Can you work these out from the model? Positions are in its coordinate system, mm. A direction names the side the tool comes from. Give positions to 0.01 mm unless a question says otherwise; leave off trailing zeros. Loops run counter-clockwise (first coordinate to the right, second up) from the corner with the lowest first, then second, coordinate; pieces in that order, holes last. Notation, with made-up numbers: (-39, -1) - (-25, -1) arc R30 cw to (-25, 38) - close; hole circle Ø1 at (-23, 28). An arc over 180 degrees is marked (long way). Answer as a JSON object with one key per item and string values.
```python
from build123d import *

# Parameters (mm, degrees)
SKETCH1_W           = 25.4
SKETCH1_H           = 50.8
SKETCH1_W_2         = 19.05
SKETCH1_H_2         = 44.45
BOSS_EXTRUDE1_DEPTH = 154.051
SKETCH2_R           = 3.175
CUT_EXTRUDE1_DEPTH  = 165.187425222
SKETCH3_R           = 3.175
CUT_EXTRUDE2_DEPTH  = 165.187425222


with BuildPart() as part:
    # Sketch1 → Boss-Extrude1 (new body)
    with BuildSketch(Plane.XY):
        with Locations((12.7, 25.4)):
            Rectangle(SKETCH1_W, SKETCH1_H)
        with Locations((12.7, 25.4)):
            Rectangle(SKETCH1_W_2, SKETCH1_H_2, mode=Mode.SUBTRACT)
    extrude(amount=BOSS_EXTRUDE1_DEPTH)

    # Sketch2 → Cut-Extrude1 (cut, through all)
    with BuildSketch(Plane(origin=(0, 50.8, 0), x_dir=(1, 0, 0), z_dir=(0, 1, 0))):
        with Locations(Location((12.7, -126.111, 0), (0, 0, 270))):
            Circle(SKETCH2_R)
        with Locations(Location((12.7, -107.061, 0), (0, 0, 270))):
            Circle(SKETCH2_R)
        with Locations(Location((12.7, -88.011, 0), (0, 0, 270))):
            Circle(SKETCH2_R)
        with Locations(Location((12.7, -27.94, 0), (0, 0, 90))):
            Circle(SKETCH2_R)
        with Locations(Location((12.7, -46.99, 0), (0, 0, 90))):
            Circle(SKETCH2_R)
        with Locations(Location((12.7, -66.04, 0), (0, 0, 90))):
            Circle(SKETCH2_R)
    extrude(amount=-CUT_EXTRUDE1_DEPTH, mode=Mode.SUBTRACT)

    # Sketch3 → Cut-Extrude2 (cut, through all)
    with BuildSketch(Plane(origin=(25.4, 0, 0), x_dir=(0, 0, -1), z_dir=(1, 0, 0))):
        with Locations(Location((-18.542, 25.4, 0), (0, 0, 90))):
            Circle(SKETCH3_R)
        with Locations(Location((-37.592, 25.4, 0), (0, 0, 90))):
            Circle(SKETCH3_R)
        with Locations(Location((-56.642, 25.4, 0), (0, 0, 90))):
            Circle(SKETCH3_R)
        with Locations(Location((-75.692, 25.4, 0), (0, 0, 90))):
            Circle(SKETCH3_R)
    extrude(amount=-CUT_EXTRUDE2_DEPTH, mode=Mode.SUBTRACT)


solid = part.part
```
1) Imagine slicing it at D-D on x = 12.7. Give the number of separate pieces and of enclosed holes in the cut face, and give its area (3 significant figures).
Check sheet entries:
{"separate pieces": "14", "enclosed holes": "0", "area": "736 mm2"}
2) If we mould it in two halves opening along X, with no side actions, what happens to faces 3 (the cylindrical face through (23.835, 27.107, 59.319)), 4 (the flat face through (13, 47.625, 76))? For each: released by +X, released by -X, zero draft, split by the parting line, or undercut.
Check sheet entries:
{"face 3": "zero draft", "face 4": "undercut"}
3) Imagine slicing it at C-C on z = 11.5. Write out the boundary of the cut face in (x, y) (3 decimals).
Check sheet entries:
{"outline": "(0, 0) - (25.4, 0) - (25.4, 50.8) - (0, 50.8) - close; hole (3.175, 3.175) - (22.225, 3.175) - (22.225, 47.625) - (3.175, 47.625) - close"}
4) I need wall thicknesses on L1, parallel to X at y = 40.5, z = 134 (3 decimals); L2, parallel to Y at x = 5.75, z = 7 (3 decimals). Which ranges of each line are inside material? Lowest first, please.
Check sheet entries:
{"L1": "0 to 3.175, 22.225 to 25.4", "L2": "0 to 3.175, 47.625 to 50.8"}
5) Imagine slicing it at A-A on z = 46.99. Write out the boundary of the cut face in (x, y) (3 decimals), and give its area (3 significant figures).
Check sheet entries:
{"outline": "(0, 0) - (9.525, 0) - (9.525, 3.175) - (3.175, 3.175) - (3.175, 47.625) - (9.525, 47.625) - (9.525, 50.8) - (0, 50.8) - close; (15.875, 0) - (25.4, 0) - (25.4, 50.8) - (15.875, 50.8) - (15.875, 47.625) - (22.225, 47.625) - (22.225, 3.175) - (15.875, 3.175) - close", "area": "403 mm2"}
6) Imagine slicing it at B-B on y = 39.5. Write out the boundary of the cut face in (x, z) (3 decimals).
Check sheet entries:
{"outline": "(0, 0) - (3.175, 0) - (3.175, 154.051) - (0, 154.051) - close; (22.225, 0) - (25.4, 0) - (25.4, 154.051) - (22.225, 154.051) - close"}
7) I'm going to push flat-ended pins straight in: P1, Ø5.5, axis at x = 12.5, z = 85.5, coming from the -Y side; P2, Ø5.5, axis at x = 12.7, z = 126.111, coming from the +Y side. Where does each tip first touch, or does it pass through?
Check sheet entries:
{"P1": "y = 0", "P2": "through"}
8) Which directions (+Z, -Z, +X, -X, +Y, -Y) give clear straight access to the entire face, cutting with the end or side of a thin tool? Please do faces 1 (the flat face through (2, 24, 0)), 2 (the flat face through (22.225, 30, 76)).
Check sheet entries:
{"face 1": "-Z, +X, -X, +Y, -Y", "face 2": "+Z, -Z"}
